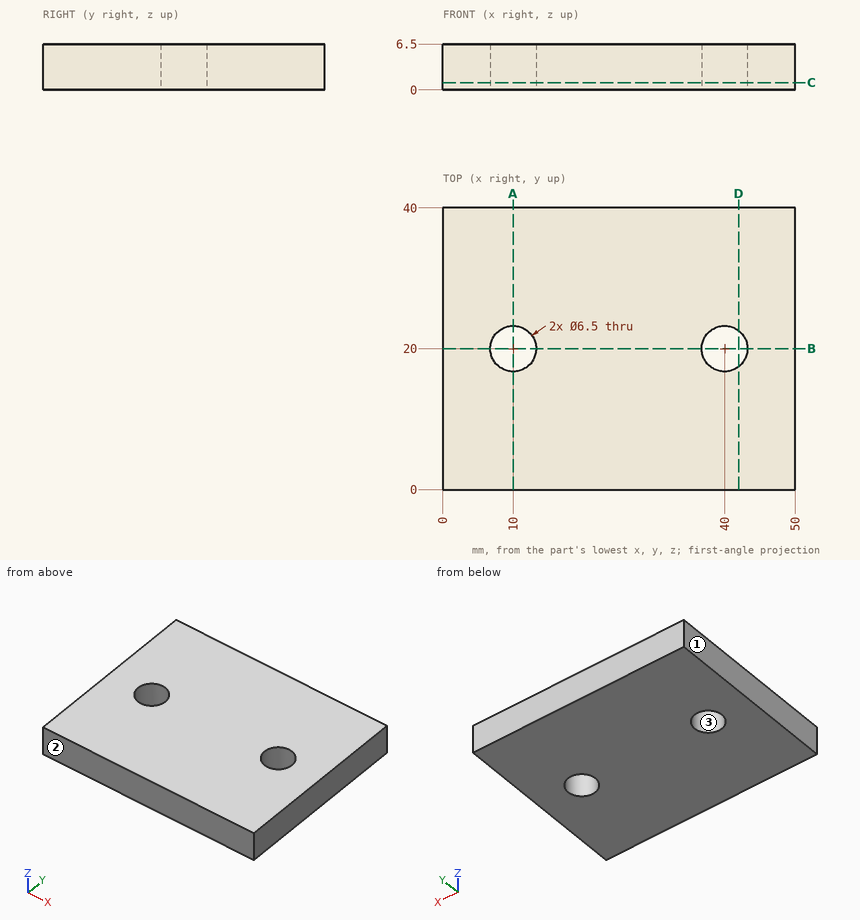
Part print with two shaded views. Sizes in mm from the minimum x, y, z corner. Coordinates: 2 decimals unless noted, no trailing zeros. Order: outer loops, then holes, each group sorted by start corner. A loop starts at its lowest first (then second) coordinate and runs counter-clockwise, first axis right, second up.
(1) Saw through at A-A, the plane x = 10. Write the cut outline in (y, z).
Solution:
outline: (0, 0) - (16.75, 0) - (16.75, 6.5) - (0, 6.5) - close; (23.25, 0) - (40, 0) - (40, 6.5) - (23.25, 6.5) - close
(2) Saw through at B-B, the plane y = 20. Write the cut outline in (x, z).
Solution:
outline: (0, 0) - (6.75, 0) - (6.75, 6.5) - (0, 6.5) - close; (13.25, 0) - (36.75, 0) - (36.75, 6.5) - (13.25, 6.5) - close; (43.25, 0) - (50, 0) - (50, 6.5) - (43.25, 6.5) - close
(3) Saw through at D-D, the plane x = 42. Write the cut outline in (y, z).
Solution:
outline: (0, 0) - (17.44, 0) - (17.44, 6.5) - (0, 6.5) - close; (22.56, 0) - (40, 0) - (40, 6.5) - (22.56, 6.5) - close
(4) Drill centre lines: L1, parallel to X at y = 20, z = 2.25; L2, parallel to Y at x = 40, z = 3; L3, parallel to X at y = 18.5, z = 4.75. Where is each one in solid material? Low to high.
Solution:
L1: x = 0 to 6.75, 13.25 to 36.75, 43.25 to 50
L2: y = 0 to 16.75, 23.25 to 40
L3: x = 0 to 7.12, 12.88 to 37.12, 42.88 to 50
(5) Saw through at C-C, the plane z = 1. Write the cut outline in (x, y), and give its area (3 significant figures).
Solution:
outline: (0, 0) - (50, 0) - (50, 40) - (0, 40) - close; hole circle Ø6.5 at (10, 20); hole circle Ø6.5 at (40, 20)
area: 1,930 mm2
(6) Mould opens along X. For the marked faces 1, 2 and 3 say: released by +X, released by -X, zero draft, split by the parting line, or undercut.
Solution:
face 1: released by -X
face 2: zero draft
face 3: undercut
